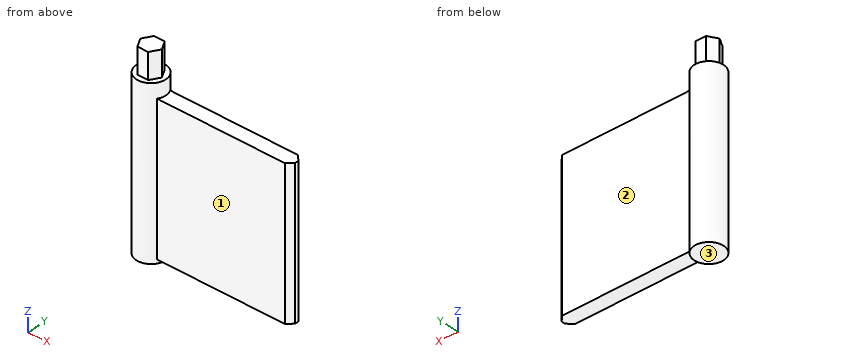
```python
from build123d import *

# Parameters (mm, degrees)
SKETCH015_W               = 40
SKETCH015_H               = 40
EXTRUDE017_DEPTH          = 2
CHAMFER_SIZE              = 1.5
EXTRUDE023_DEPTH          = 7
SKETCH014_R               = 4
EXTRUDE016_DEPTH          = 45
FUSION007_PLACEMENT_ANGLE = 180


with BuildPart() as chamfer_body:
    # Sketch015 (on Extrude) → Extrude017 (new body, symmetric)
    with BuildSketch(Plane.XZ):
        with Locations((-20, 24)):
            Rectangle(SKETCH015_W, SKETCH015_H)
    extrude(amount=EXTRUDE017_DEPTH, both=True)

    # Chamfer
    chamfer_edges = [chamfer_body.edges().sort_by_distance(p)[0] for p in [
        (-40, 2, 24),
        (-40, -2, 24),
    ]]
    chamfer(chamfer_edges, length=CHAMFER_SIZE)


with BuildPart() as extrude023:
    # Sketch018 → Extrude023 (new body)
    with BuildSketch(Plane.XY):
        Polygon((-1.475, 2.554775), (1.475, 2.554775), (2.95, 0), (1.475, -2.554775), (-1.475, -2.554775), (-2.95, 0), align=None)
    extrude(amount=-EXTRUDE023_DEPTH)


with BuildPart() as flap:
    # Sketch014 → Extrude016 (new body)
    with BuildSketch(Plane.XY):
        Circle(SKETCH014_R)
    extrude(amount=EXTRUDE016_DEPTH)

    # Fusion007: union Chamfer body, Extrude023
    add(chamfer_body.part)
    add(extrude023.part)


with BuildPart() as flap_1:
    # Fusion007 placement: moved
    add(flap.part.rotate(Axis((0, 0, 0), (0, 1, 0)), FUSION007_PLACEMENT_ANGLE))


solid = flap_1.part
```
Model file for the job. Use its own axes, mm. Face numbers are marked on the shaded views. A direction names the side the tool comes from. Round coordinates to 2 decimals unless told otherwise and drop trailing zeros. Order: outer loops, then holes, each group sorted by start corner. A loop starts at its lowest first (then second) coordinate and runs counter-clockwise, first axis right, second up. Notation, with made-up numbers: (-11, 2.25) -> (11, 2.25) arc R27 cw to (11, 20.25) -> close; hole circle Ø8 at (73, -10.5). An arc over 180 degrees is marked (long way). Use one line per item in the form item = value.
Item 1: Drill centre lines: line 1 (Y direction, x = 37, z = -36.5); line 2 (Z direction, x = 33.5, y = 1); line 3 (X direction, y = 1, z = -24.5). Where is each one in solid material? Low to high.
Returned:
line_1 = -2 to 2
line_2 = -44 to -4
line_3 = -3.87 to 39.5
Item 2: Tool access for the marked faces 1, 2 and 3: list every direction of +Z, -Z, +X, -X, +Y, -Y with a clear straight run to the whole face (end or side of a thin tool).
Returned:
face_1 = +Z, -Z, +X, -Y
face_2 = +Z, -Z, +X, +Y
face_3 = -Z, +X, -X, +Y, -Y
Item 3: Flat gauge pins, fed straight in: pin 1 Ø2.5 at (x, z) = (0, 4.5) entering from +Y; pin 2 Ø0.9 at (x, z) = (0.5, 3) entering from -Y; pin 3 Ø4 at (x, y) = (27, 2.5) entering from +Z. Where does each tip first touch, or does it go through?
Returned:
pin_1 = 2.55
pin_2 = -2.55
pin_3 = -4
Item 4: Cut at A-A, the plane x = 0. Write the cut outline in (y, z), and give its area (3 significant figures).
Returned:
outline = (-4, -45) -> (4, -45) -> (4, 0) -> (2.55, 0) -> (2.55, 7) -> (-2.55, 7) -> (-2.55, 0) -> (-4, 0) -> close
area = 396 mm^2
Item 5: Cut at B-B, the plane z = -19.5. Write the cut outline in (x, y), and give its area (3 significant figures).
Returned:
outline = (3.46, -2) -> (38.5, -2) -> (40, -0.5) -> (40, 0.5) -> (38.5, 2) -> (3.46, 2) arc R4 ccw (long way) to start
area = 193 mm^2
Item 6: Cut at C-C, the plane x = 10.5. Write the cut outline in (y, z).
Returned:
outline = (-2, -44) -> (2, -44) -> (2, -4) -> (-2, -4) -> close
